Here's how the part is built. I have some questions about the finished solid (model axes, mm). Face numbers are marked on the shaded views. A direction names the side the tool comes from. Round coordinates to 2 decimals unless told otherwise and drop trailing zeros. Loops run counter-clockwise (first coordinate to the right, second up) from the corner with the lowest first, then second, coordinate; pieces in that order, holes last. Notation, with made-up numbers: M 43,63.5 L 85,63.5 A32 ccw 85,98.5 Z; hole C -35.75,-32.5 d2. An arc over 180 degrees is marked long. Answer as a JSON object with one key per item and string values.
from build123d import *

# Parameters (mm, degrees)
SKETCH1_R           = 6.475
BOSS_EXTRUDE1_DEPTH = 58.75
SKETCH2_R           = 2.5
BOSS_EXTRUDE2_DEPTH = 2
BOSS_EXTRUDE3_DEPTH = 8.5
BOSS_EXTRUDE4_DEPTH = 20


with BuildPart() as part:
    # Sketch1 → Boss-Extrude1 (new body)
    with BuildSketch(Plane.XY):
        with Locations(Location((0, 0, 0), (0, 0, 180))):
            Circle(SKETCH1_R)
    extrude(amount=BOSS_EXTRUDE1_DEPTH)

    # Sketch2 → Boss-Extrude2 (add)
    with BuildSketch(Plane.XY.offset(58.75)):
        Circle(SKETCH2_R)
    extrude(amount=BOSS_EXTRUDE2_DEPTH)

    # Sketch3 → Boss-Extrude3 (add)
    with BuildSketch(Plane.XY.offset(60.75)):
        with BuildLine():
            Line((0, 1.25), (-0.829156198, 1.25))
            ThreePointArc((-0.829156198, 1.25), (-1.436140662, -0.433012702), (0, -1.5))
            Line((0, -1.5), (0, 1.25))
        make_face()
        with BuildLine():
            Line((0.829156198, 1.25), (0, 1.25))
            Line((0, 1.25), (0, -1.5))
            ThreePointArc((0, -1.5), (1.060660172, -1.060660172), (1.5, 0))
            ThreePointArc((1.5, 0), (1.321691018, 0.709318583), (0.829156198, 1.25))
        make_face()
    extrude(amount=BOSS_EXTRUDE3_DEPTH)

    # Sketch4 → Boss-Extrude4 (add)
    with BuildSketch(Plane(origin=(0, 0, 0), x_dir=(-1, 0, 0), z_dir=(0, 0, -1))):
        with BuildLine():
            Line((-3.4, 3.775), (3.4, 3.775))
            ThreePointArc((3.4, 3.775), (3.9, 3.275), (3.4, 2.775))
            Line((3.4, 2.775), (-3.4, 2.775))
            ThreePointArc((-3.4, 2.775), (-3.9, 3.275), (-3.4, 3.775))
        make_face()
    extrude(amount=BOSS_EXTRUDE4_DEPTH)


solid = part.part
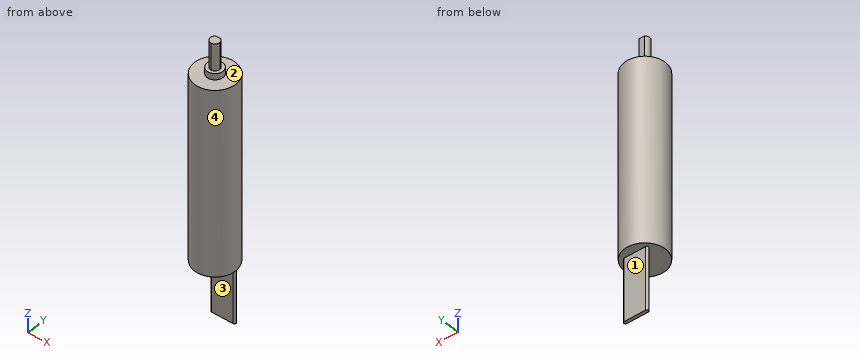
Item 1: I'm going to push flat-ended pins straight in: pin 1 Ø1 at (x, z) = (3.5, 29) entering from -Y; pin 2 Ø5 at (x, z) = (-4.5, 52) entering from +Y; pin 3 Ø1.5 at (x, z) = (-2, -5.5) entering from +Y (3 decimals); pin 4 Ø3 at (x, y) = (0, 2.5) entering from +Z. Where does each tip first touch, or does it pass through?
Resolved:
{"pin 1": "y = -5.74", "pin 2": "y = 6.16", "pin 3": "y = 3.775", "pin 4": "z = 69.25"}
Item 2: I want a section at A-A, the plane z = -14. Please give me the cut outline in (x, y) (3 decimals).
Resolved:
{"outline": "M -3.4,2.775 L 3.4,2.775 A0.5 ccw 3.4,3.775 L -3.4,3.775 A0.5 ccw Z"}
Item 3: I want a section at C-C, the plane z = 12. Please give me the cut outline in (x, y) (3 decimals), then the cut area to 3 significant figures.
Resolved:
{"outline": "C 0,0 d12.95", "area": "132 mm²"}
Item 4: On a 3-axis mill with a long thin cutter (end or side, diameter ignored), from which of +Z, -Z, +X, -X, +Y, -Y can I reach the whole of each face in a straight line? I mean the marked faces 1, 2, 3 and 4. Say none if no direction works.
Resolved:
{"face 1": "-Z, +X, -X, +Y", "face 2": "+Z", "face 3": "-Z, +X, -X, -Y", "face 4": "+Z, -Z"}
Item 5: I want a section at B-B, the plane x = 5.5. Please give me the cut outline in (y, z), then the cut area to 3 significant figures.
Resolved:
{"outline": "M -3.42,0 L 3.42,0 L 3.42,58.75 L -3.42,58.75 Z", "area": "401 mm²"}
Item 6: Please list where these lines run through material, in increasing order: probe 1 along Z at (x, y) = (-0.5, 4.5); probe 2 along Z at (x, y) = (1.5, 3.25); probe 3 along Y at (x, z) = (3, -12.5) (3 decimals). Write a range as from..to.
Resolved:
{"probe 1": "0..58.75", "probe 2": "-20..58.75", "probe 3": "2.775..3.775"}
